```python
from build123d import *

# Parameters (mm, degrees)
F1_DEPTH = 50
F5_D     = 18
F6_D     = 14
F7_D     = 14


with BuildPart() as f1:
    # F0 (on Front) → F1 (new body)
    with BuildSketch(Plane.XZ):
        with BuildLine():
            Line((0, 15), (0, 0))
            Line((0, 0), (32, 0))
            ThreePointArc((32, 0), (48.2634559673, 6.7365440327), (55, 23))
            Line((55, 23), (55, 37))
            ThreePointArc((55, 37), (57.3431457505, 42.6568542495), (63, 45))
            Line((63, 45), (131, 45))
            ThreePointArc((131, 45), (136.6568542495, 42.6568542495), (139, 37))
            Line((139, 37), (139, 23))
            ThreePointArc((139, 23), (145.7365440327, 6.7365440327), (162, 0))
            Line((162, 0), (194, 0))
            Line((194, 0), (194, 15))
            Line((194, 15), (162, 15))
            ThreePointArc((162, 15), (156.3431457505, 17.3431457505), (154, 23))
            Line((154, 23), (154, 37))
            ThreePointArc((154, 37), (147.2634559673, 53.2634559673), (131, 60))
            Line((131, 60), (63, 60))
            ThreePointArc((63, 60), (46.7365440327, 53.2634559673), (40, 37))
            Line((40, 37), (40, 23))
            ThreePointArc((40, 23), (37.6568542495, 17.3431457505), (32, 15))
            Line((32, 15), (0, 15))
        make_face()
    extrude(amount=F1_DEPTH)

    # F5 (through all)
    with Locations(Plane(origin=(0, 0, 45), x_dir=(1, 0, 0), z_dir=(0, 0, -1))):
        with Locations((97, 25)):
            Hole(F5_D / 2)

    # F6 (through all)
    with Locations(Plane(origin=(0, 0, 0), x_dir=(1, 0, 0), z_dir=(0, 0, -1))):
        with Locations((17, 25)):
            Hole(F6_D / 2)

    # F7 (through all)
    with Locations(Plane(origin=(0, 0, 0), x_dir=(1, 0, 0), z_dir=(0, 0, -1))):
        with Locations((177, 25)):
            Hole(F7_D / 2)


solid = f1.part
```
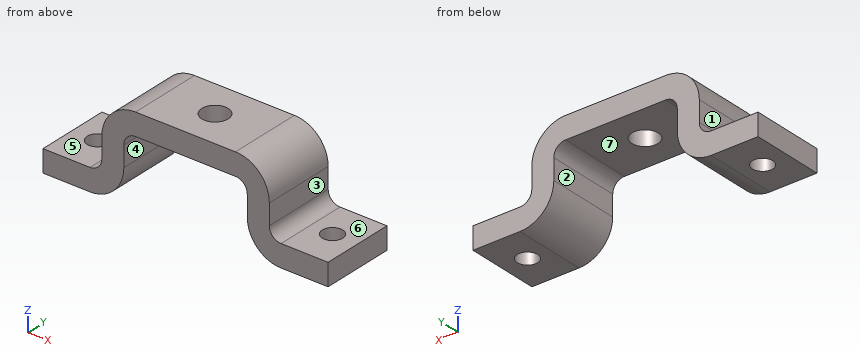
Design review of the part built by this model. Coordinates are the model's own, in mm. Face numbers are marked on the shaded views. A direction names the side the tool comes from. Coordinates: 2 decimals unless noted, no trailing zeros. Order: outer loops, then holes, each group sorted by start corner. A loop starts at its lowest first (then second) coordinate and runs counter-clockwise, first axis right, second up.
1) Mouldability with a two-part tool opening along X and no side actions: class the marked faces 1, 2, 3 and 4 as +X half, -X half, draft (parallel to the pull), parting line (faces both ways), or undercut.
2) Clearance check with flat-ended pins moving along their axes: pin 1 (9.5 mm diameter, centred on x = 180.5, y = -25.5, fed in from +Z); pin 2 (8.5 mm diameter, centred on x = 17, y = -25, fed in from +Z); pin 3 (1 mm diameter, centred on y = -8.5, z = 21.5, fed in from -X); pin 4 (15.5 mm diameter, centred on y = -14, z = 30, fed in from +X). State where each tip first meets the part, or that it passes through.
3) Take a section at B-B, the plane y = -27.5. State how many separate pieces and enclosed holes the cut face has, and give its area (3 significant figures).
4) For the marked faces 5, 6 and 7, list the 3-axis set-ups (+Z, -Z, +X, -X, +Y, -Y) from which the entire face can be reached by the end or side of a thin tool; tool diameter is ignored.
5) Take a section at A-A, the plane x = 97. Give the boundary of the cut face in (y, z), and give its area (3 significant figures).
6) Wall thickness on line 1 along X through (y, z) = (-6, 33); line 2 along X through (y, z) = (-25, 11); line 3 along Y through (x, z) = (17, 4.5): over which ranges is each line inside the solid? List them lowest first.
7) Take a section at C-C, the plane z = 54. Give the boundary of the cut face in (x, y), and give its area (3 significant figures).
8) Take a section at D-D, the plane x = 177. Give the boundary of the cut face in (y, z).
Returned:
1. face 1: -X half
1. face 2: undercut
1. face 3: +X half
1. face 4: undercut
2. pin 1: stops at z = 15
2. pin 2: passes through
2. pin 3: stops at x = 39.75
2. pin 4: stops at x = 154.04
3. separate pieces: 4
3. enclosed holes: 0
3. area: 3,210 mm2
4. face 5: +Z, -X, +Y, -Y
4. face 6: +Z, +X, +Y, -Y
4. face 7: -Z, +Y, -Y
5. outline: (-50, 45) - (-34, 45) - (-34, 60) - (-50, 60) - close; (-16, 45) - (0, 45) - (0, 60) - (-16, 60) - close
5. area: 480 mm2
6. line 1: x = 40 to 55, 139 to 154
6. line 2: x = 0 to 10, 24 to 51.62, 142.38 to 170, 184 to 194
6. line 3: y = -50 to -32, -18 to 0
7. outline: (47.51, -50) - (146.49, -50) - (146.49, 0) - (47.51, 0) - close; hole circle Ø18 at (97, -25)
7. area: 4,690 mm2
8. outline: (-50, 0) - (-32, 0) - (-32, 15) - (-50, 15) - close; (-18, 0) - (0, 0) - (0, 15) - (-18, 15) - close
